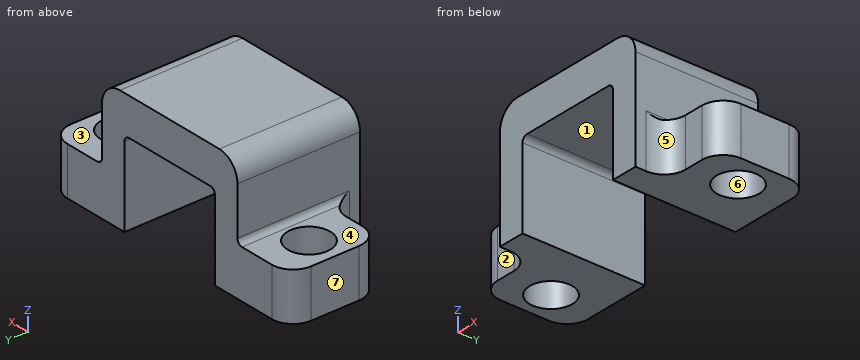
```python
from build123d import *

# Parameters (mm, degrees)
F0_W     = 26.6
F0_H     = 11.5
F1_DEPTH = 11.5
F2_W     = 5.8
F2_H     = 7
F2_W_2   = 10
F2_H_2   = 8
F3_DEPTH = 11.501
F4_W     = 5.8
F4_H     = 3
F4_R     = 2
F5_DEPTH = 4.501
F6_W     = 5.8
F6_H     = 3
F6_R     = 2
F7_DEPTH = 4.501
F8_R     = 2
F9_R     = 0.5


with BuildPart() as f1:
    # F0 (on Top) → F1 (new body)
    with BuildSketch(Plane.XY):
        Rectangle(F0_W, F0_H)
    extrude(amount=F1_DEPTH)

    # F2 (on face) → F3 (cut, through all)
    with BuildSketch(Plane.XZ.offset(5.75)):
        with Locations((-10.4, 8)):
            Rectangle(F2_W, F2_H)
        with Locations((10.4, 8)):
            Rectangle(F2_W, F2_H)
        with Locations((0, 4)):
            Rectangle(F2_W_2, F2_H_2)
    extrude(amount=-F3_DEPTH, mode=Mode.SUBTRACT)

    # F4 (on face) → F5 (cut, through all)
    with BuildSketch(Plane.XY.offset(4.5)):
        with Locations((-10.4, -4.25)):
            Rectangle(F4_W, F4_H)
        with Locations((-10.4, 1.5)):
            Circle(F4_R)
    extrude(amount=-F5_DEPTH, mode=Mode.SUBTRACT)

    # F6 (on face) → F7 (cut, through all)
    with BuildSketch(Plane.XY.offset(4.5)):
        with Locations((10.4, -4.25)):
            Rectangle(F6_W, F6_H)
        with Locations((10.3, 1.5)):
            Circle(F6_R)
    extrude(amount=-F7_DEPTH, mode=Mode.SUBTRACT)

    # F8
    f8_edges = [f1.edges().sort_by_distance(p)[0] for p in [
        (-7.5, 0, 11.5),
        (7.5, 0, 11.5),
        (-13.3, -2.75, 2.25),
        (-13.3, 5.75, 2.25),
        (-7.5, -2.75, 2.25),
        (13.3, 5.75, 2.25),
        (13.3, -2.75, 2.25),
        (7.5, -2.75, 2.25),
    ]]
    fillet(f8_edges, radius=F8_R)

    # F9
    f9_edges = [f1.edges().sort_by_distance(p)[0] for p in [
        (-7.5, 1.5, 4.5),
        (7.5, 1.5, 4.5),
        (-5, 0, 8),
        (5, 0, 8),
    ]]
    fillet(f9_edges, radius=F9_R)


solid = f1.part
```
Model file for the job. Use its own axes, mm. Face numbers are marked on the shaded views. A direction names the side the tool comes from. Round coordinates to 2 decimals unless told otherwise and drop trailing zeros. Write each loop counter-clockwise with the first axis right and the second up, starting at its lowest first coordinate (ties: lowest second). Pieces come first, ordered by that corner, then holes. Notation, with made-up numbers: (-3, 76) - (40, 76) arc R19 ccw to (40, 94) - close; hole circle Ø1 at (1.25, 2.5). An arc over 180 degrees is marked (long way). One line per item, written item: value.
(1) Drop flat-ended pins along their axis: P1, Ø1.5, axis at y = -1, z = 8.5, coming from the +X side; P2, Ø6, axis at x = 11, y = 3, coming from the +Z side; P3, Ø2, axis at x = -10, z = 2, coming from the -Y side. Give the stop position or say it passes through.
Values follow:
P1: stops at x = 7.5
P2: stops at z = 4.5
P3: stops at y = -2.81
(2) Two-plate mould, pull along Y, no slides. Class the marked faces 5, 6 and 7: pulls with the +Y half, pulls with the -Y half, needs draft (parallel to the pull), parting line crosses it, or undercut.
Values follow:
face 5: pulls with the -Y half
face 6: undercut
face 7: needs draft
(3) Cut at C-C, the plane x = 10.3. Give the cut face in (y, z), plus the area to 4 significant figures.
Values follow:
outline: (-2.75, 0) - (-0.5, 0) - (-0.5, 4.5) - (-2.75, 4.5) - close; (3.5, 0) - (5.75, 0) - (5.75, 4.5) - (3.5, 4.5) - close
area: 20.25 mm²
(4) 3-axis set-ups, long thin cutter, end or side, ignore diameter. For the marked faces 1, 2, 3 and 4: which of +Z, -Z, +X, -X, +Y, -Y reach the whole face in a straight line?
Values follow:
face 1: -Z, +Y, -Y
face 2: +Z, -Z, -X, -Y
face 3: +Z, +X, +Y, -Y
face 4: +Z, -X, +Y, -Y
(5) Cut at B-B, the plane y = 1.5. Give the cut face in (x, z), plus the area to 3 significant figures.
Values follow:
outline: (-13.3, 0) - (-12.4, 0) - (-12.4, 4.5) - (-13.3, 4.5) - close; (-8.4, 0) - (-5, 0) - (-5, 7.5) arc R0.5 cw to (-4.5, 8) - (4.5, 8) arc R0.5 cw to (5, 7.5) - (5, 0) - (8.3, 0) - (8.3, 4.5) - (8, 4.5) arc R0.5 cw to (7.5, 5) - (7.5, 9.5) arc R2 ccw to (5.5, 11.5) - (-5.5, 11.5) arc R2 ccw to (-7.5, 9.5) - (-7.5, 5) arc R0.5 cw to (-8, 4.5) - (-8.4, 4.5) - close; (12.3, 0) - (13.3, 0) - (13.3, 4.5) - (12.3, 4.5) - close
area: 107 mm²
(6) Cut at D-D, the plane z = 5.5. Give the cut face in (x, y).
Values follow:
outline: (-7.5, -5.75) - (-5, -5.75) - (-5, 5.75) - (-7.5, 5.75) - close; (5, -5.75) - (7.5, -5.75) - (7.5, 5.75) - (5, 5.75) - close
(7) Wall check: probe 1 along X at (y, z) = (2.25, 6.25); probe 2 along Y at (x, z) = (-10.4, 1.1); probe 3 along Z at (x, y) = (-8.25, -3). Give the ranges that are in metal, low to high.
Values follow:
probe 1: x = -7.5 to -5, 5 to 7.5
probe 2: y = -2.75 to -0.5, 3.5 to 5.75
probe 3: z = 0 to 4.5
(8) Cut at A-A, the plane z = 2. Give the cut face in (x, y).
Values follow:
outline: (-13.3, -0.75) arc R2 ccw to (-11.3, -2.75) - (-9.5, -2.75) arc R2 cw to (-7.5, -4.75) - (-7.5, -5.75) - (-5, -5.75) - (-5, 5.75) - (-11.3, 5.75) arc R2 ccw to (-13.3, 3.75) - close; (5, -5.75) - (7.5, -5.75) - (7.5, -4.75) arc R2 cw to (9.5, -2.75) - (11.3, -2.75) arc R2 ccw to (13.3, -0.75) - (13.3, 3.75) arc R2 ccw to (11.3, 5.75) - (5, 5.75) - close; hole circle Ø4 at (-10.4, 1.5); hole circle Ø4 at (10.3, 1.5)
